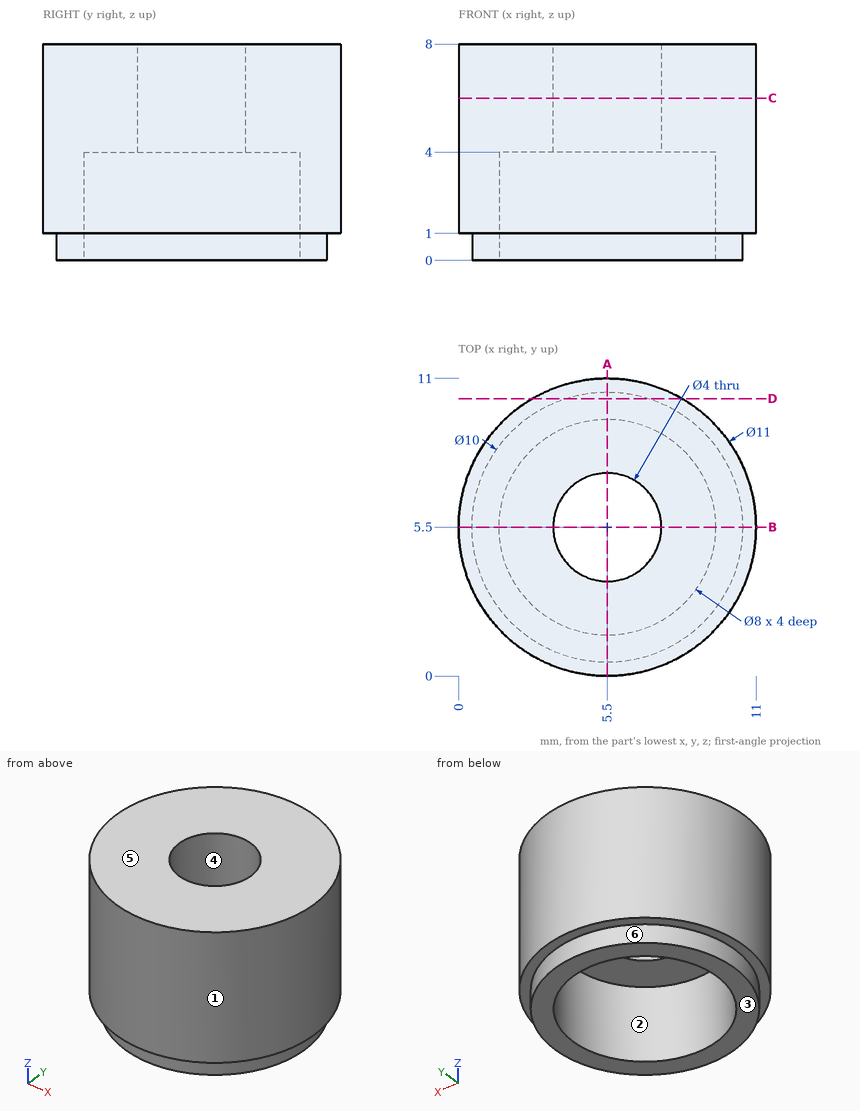
Geometry check sheet. Reference: drawing and pictorial views, mm from the part's lowest x, y, z. A direction names the side the tool comes from. Coordinates: 2 decimals unless noted, no trailing zeros. Loops run counter-clockwise (first coordinate to the right, second up) from the corner with the lowest first, then second, coordinate; pieces in that order, holes last. Notation, with made-up numbers: (53, 34) - (89, 34) arc R25 ccw to (89, 50) - close; hole circle Ø2 at (43, -24.75). An arc over 180 degrees is marked (long way). Return JSON: item names as keys, results as strings.
1. Section check A-A, the plane x = 5.5. Record the boundary of the cut face in (y, z).
Established:
{"outline": "(0, 1) - (0.5, 1) - (0.5, 0) - (1.5, 0) - (1.5, 4) - (3.5, 4) - (3.5, 8) - (0, 8) - close; (7.5, 4) - (9.5, 4) - (9.5, 0) - (10.5, 0) - (10.5, 1) - (11, 1) - (11, 8) - (7.5, 8) - close"}
2. Mould release check, pull along X, two halves, no side actions. Record for the marked faces 1, 2, 3 and 4: +X half, -X half, draft (parallel to the pull), parting line (faces both ways), or undercut.
Established:
{"face 1": "parting line", "face 2": "undercut", "face 3": "draft", "face 4": "undercut"}
3. Section check D-D, the plane y = 10.25. Record the boundary of the cut face in (x, z), then the cut area to 3 significant figures.
Established:
{"outline": "(2.73, 1) - (3.94, 1) - (3.94, 0) - (7.06, 0) - (7.06, 1) - (8.27, 1) - (8.27, 8) - (2.73, 8) - close", "area": "41.9 mm2"}
4. Thickness scan on L1, parallel to Y at x = 5.5, z = 2.25; L2, parallel to Y at x = 5.5, z = 6. Record the ranges inside material, lowest first.
Established:
{"L1": "y = 0 to 1.5, 9.5 to 11", "L2": "y = 0 to 3.5, 7.5 to 11"}
5. Section check C-C, the plane z = 6. Record the boundary of the cut face in (x, y).
Established:
{"outline": "circle Ø11 at (5.5, 5.5); hole circle Ø4 at (5.5, 5.5)"}
6. Tool access check on the marked faces 5 and 6. Record the directions out of +Z, -Z, +X, -X, +Y, -Y that give a thin tool (end or side, any length) a straight path to the whole face; none if there is none.
Established:
{"face 5": "+Z, +X, -X, +Y, -Y", "face 6": "-Z"}
7. Go/stop test with flat-tipped pins: pin 1 (1.5 mm diameter, centred on x = 6.5, z = 7, fed in from +Y); pin 2 (3 mm diameter, centred on y = 2.5, z = 2.5, fed in from -X); pin 3 (1 mm diameter, centred on x = 3.5, z = 7, fed in from +Y). Record where each tip stops, or that it passes through.
Established:
{"pin 1": "stops at y = 10.99", "pin 2": "stops at x = 0.21", "pin 3": "stops at y = 10.79"}
